Source: CAD feature listing. Evaluate the final solid. Frame: model axes, mm. Face numbers are marked on the shaded views. A direction names the side the tool comes from. Coordinates: 2 decimals unless noted, no trailing zeros. Loops run counter-clockwise (first coordinate to the right, second up) from the corner with the lowest first, then second, coordinate; pieces in that order, holes last. Notation, with made-up numbers: (38, 75) - (42, 75) arc R19 cw to (42, 101) - close; hole circle Ø9 at (1.5, 57). An arc over 180 degrees is marked (long way). Use one line per item in the form item = value. Start each with the question number.
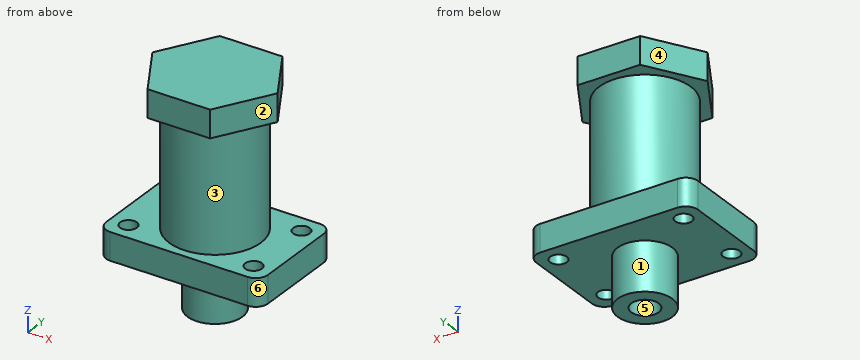
from build123d import *

# Parameters (mm, degrees)
F1_DEPTH  = 57.15
F2_R      = 95.25
F3_DEPTH  = 250.825
F5_DEPTH  = 57.15
F7_D      = 34.925
F8_R      = 57.15
F9_DEPTH  = 101.6
F11_D     = 57.15
F11_DEPTH = 406.4
F11_TIP   = 17.1695921887


with BuildPart() as f1:
    # F0 (on Top) → F1 (new body)
    with BuildSketch(Plane.XY):
        with BuildLine():
            Line((142.875, 112.7125), (-142.875, 112.7125))
            ThreePointArc((-142.875, 112.7125), (-160.8355122421, 105.2730122421), (-168.275, 87.3125))
            Line((-168.275, 87.3125), (-168.275, -87.3125))
            ThreePointArc((-168.275, -87.3125), (-160.8355122421, -105.2730122421), (-142.875, -112.7125))
            Line((-142.875, -112.7125), (142.875, -112.7125))
            ThreePointArc((142.875, -112.7125), (160.8355122421, -105.2730122421), (168.275, -87.3125))
            Line((168.275, -87.3125), (168.275, 87.3125))
            ThreePointArc((168.275, 87.3125), (160.8355122421, 105.2730122421), (142.875, 112.7125))
        make_face()
    extrude(amount=F1_DEPTH)

    # F2 (on face) → F3 (join)
    with BuildSketch(Plane.XY.offset(57.15)):
        Circle(F2_R)
    extrude(amount=F3_DEPTH)

    # F4 (on face) → F5 (join)
    with BuildSketch(Plane.XY.offset(307.975)):
        Polygon((65.11400916, 112.7807721496), (-65.11400916, 112.7807721496), (-130.2280183199, 0), (-65.11400916, -112.7807721496), (65.11400916, -112.7807721496), (130.2280183199, 0), align=None)
    extrude(amount=F5_DEPTH)

    # F7 (through all)
    with Locations(Plane(origin=(0, 0, 0), x_dir=(1, 0, 0), z_dir=(0, 0, -1))):
        with Locations((-130.175, 74.676), (-130.175, -74.676), (130.175, -74.676), (130.175, 74.676)):
            Hole(F7_D / 2)

    # F8 (on face) → F9 (join)
    with BuildSketch(Plane(origin=(0, 0, 0), x_dir=(1, 0, 0), z_dir=(0, 0, -1))):
        Circle(F8_R)
    extrude(amount=F9_DEPTH)

    # F11
    with Locations(Plane(origin=(0, 0, -101.6), x_dir=(1, 0, 0), z_dir=(0, 0, -1))):
        with Locations((0, 0)):
            Hole(F11_D / 2, depth=F11_DEPTH)
            with Locations((0, 0, -(F11_DEPTH + F11_TIP / 2))):  # 118° drill point
                Cone(0, F11_D / 2, F11_TIP, mode=Mode.SUBTRACT)


solid = f1.part
(1) Mould query, pull axis X, two halves, no side actions, for the marked faces 4, 5 and 6. Classes: +X half, -X half, draft (parallel to the pull), parting line (faces both ways), or undercut.
(2) Contact query for flat-ended pins moving along their axis: pin 1 (5 mm diameter, centred on y = -79, z = 144, fed in from -X); pin 2 (8 mm diameter, centred on x = 105, y = -69.5, fed in from -Z); pin 3 (10 mm diameter, centred on y = 39, z = -1.5, fed in from -X) (3 decimals); pin 4 (1.5 mm diameter, centred on x = -85.5, z = 201.5, fed in from +Y). Output: stop coordinate, or through.
(3) Access query for the marked faces 1, 2 and 3. Directions: +Z, -Z, +X, -X, +Y, -Y. A direction counts if a zero-diameter tool reaches every point of the face in a straight line with its end or side. Return the directions, or none.
(4) Material intervals for line 1 (X direction, y = -0.5, z = 60); line 2 (Z direction, x = 93.5, y = 52.5) (3 decimals); line 3 (X direction, y = -63, z = 28.5) (3 decimals), sorted ascending.
(5) Cut plane B-B, the plane z = -6. Output: boundary loops of the cut face in (x, y) (3 decimals), plus the area to 3 significant figures.
(6) Cut plane D-D, the plane y = 40.5. Output: boundary loops of the cut face in (x, z) (3 decimals).
Recorded:
q1.face_4 = -X half
q1.face_5 = undercut
q1.face_6 = +X half
q2.pin_1 = -56.75
q2.pin_2 = 0
q2.pin_3 = -168.275
q2.pin_4 = 43.47
q3.face_1 = -Z
q3.face_2 = +Z, +X, -Y
q3.face_3 = none
q4.line_1 = -95.25 to -28.57, 28.57 to 95.25
q4.line_2 = 0 to 57.15, 307.975 to 365.125
q4.line_3 = -168.275 to -143.16, -117.19 to 117.19, 143.16 to 168.275
q5.outline = circle Ø114.3 at (0, 0); hole circle Ø57.15 at (0, 0)
q5.area = 7,700 mm²
q6.outline = (-168.275, 0) - (-40.322, 0) - (-40.322, -101.6) - (40.322, -101.6) - (40.322, 0) - (168.275, 0) - (168.275, 57.15) - (86.211, 57.15) - (86.211, 307.975) - (106.845, 307.975) - (106.845, 365.125) - (-106.845, 365.125) - (-106.845, 307.975) - (-86.211, 307.975) - (-86.211, 57.15) - (-168.275, 57.15) - close
